Job drawing, mm, ordinate dimensions from the low corner. One solid piece. Give positions to 0.01 mm unless a question says otherwise; leave off trailing zeros. Loops run counter-clockwise (first coordinate to the right, second up) from the corner with the lowest first, then second, coordinate; pieces in that order, holes last. Notation, with made-up numbers: M -20.75,11 L 13.25,11 A22 cw 13.25,32 Z; hole C -31.75,39 d4. An arc over 180 degrees is marked long. One line per question, with ' | ' between items.
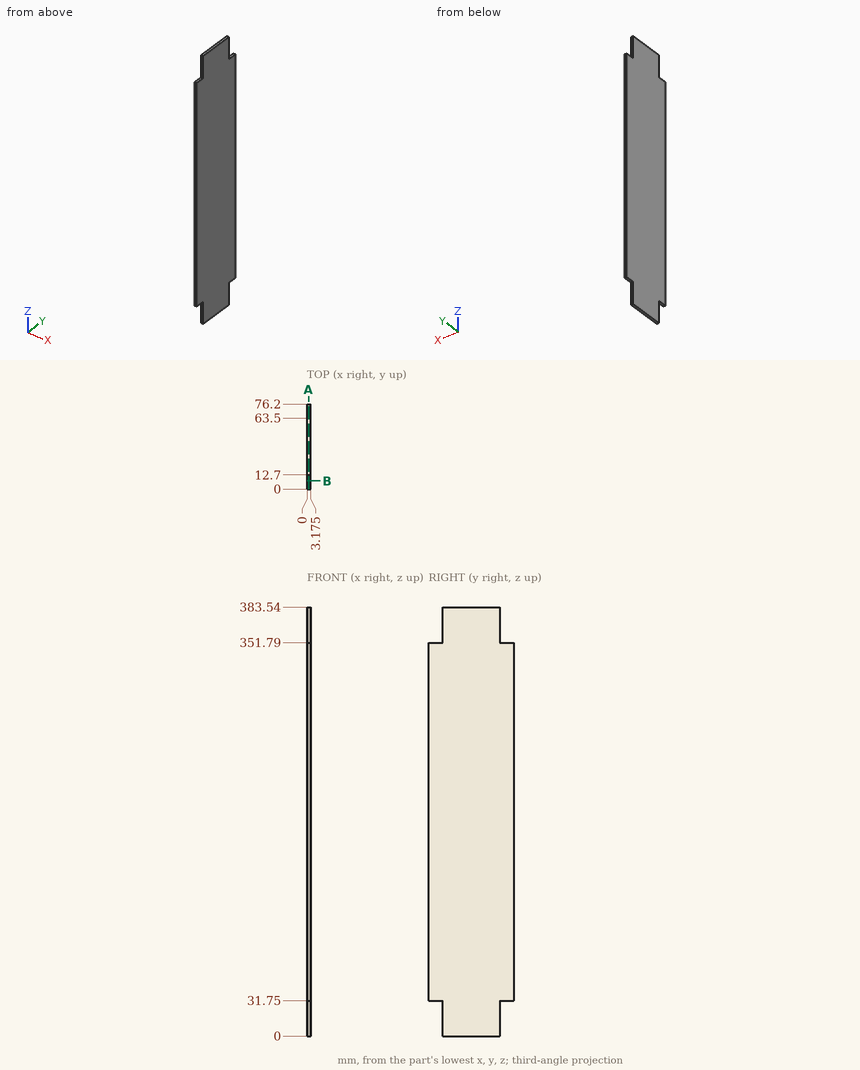
Item 1: Drop flat-ended pins along their axis: P1, Ø1, axis at x = 2, z = 364, coming from the -Y side; P2, Ø1.6, axis at x = 2.5, y = 71, coming from the -Z side. Give the stop position or say it passes through.
Conclusion:
P1: y = 12.7 | P2: z = 31.75
Item 2: Saw through at B-B on y = 7.5. Give the cut face in (x, z) (3 decimals), and give its area (3 significant figures).
Conclusion:
outline: M 0,31.75 L 3.175,31.75 L 3.175,351.79 L 0,351.79 Z | area: 1,020 mm²
Item 3: Saw through at A-A on x = 1.35. Give the cut face in (y, z), and give its area (3 significant figures).
Conclusion:
outline: M 0,31.75 L 12.7,31.75 L 12.7,0 L 63.5,0 L 63.5,31.75 L 76.2,31.75 L 76.2,351.79 L 63.5,351.79 L 63.5,383.54 L 12.7,383.54 L 12.7,351.79 L 0,351.79 Z | area: 27,600 mm²
Item 4: Drill centre lines: line 1 along Y through (x, z) = (1.8, 18); line 2 along Z through (x, y) = (1.6, 64). Where is each one in solid material? Low to high. Write a range as [from, to].
Conclusion:
line 1: [12.7, 63.5] | line 2: [31.75, 351.79]
